Model file for the job. Use its own axes, mm. A direction names the side the tool comes from. Give positions to 0.01 mm unless a question says otherwise; leave off trailing zeros. Write each loop counter-clockwise with the first axis right and the second up, starting at its lowest first coordinate (ties: lowest second). Pieces come first, ordered by that corner, then holes. Notation, with made-up numbers: M 54,31.25 L 89,31.25 A32 cw 89,57.25 Z; hole C -11,50 d3. An arc over 180 degrees is marked long. Answer as a JSON object with one key per item and string values. Group by question number.
```python
from build123d import *

# Parameters (mm, degrees)
BOSS_EXTRUDE1_DEPTH = 9.5
SKETCH3_R           = 2.75
SKETCH3_R_2         = 1.25
CUT_EXTRUDE1_DEPTH  = 19.054661658


with BuildPart() as part:
    # Sketch2 → Boss-Extrude1 (new body, symmetric)
    with BuildSketch(Plane.XY):
        with BuildLine():
            Line((-37.204062484, 20.661621188), (-37.204062484, 2.661621188))
            ThreePointArc((-37.204062484, 2.661621188), (-35.886988122, -0.518077598), (-32.707289335, -1.83515196))
            Line((-32.707289335, -1.83515196), (-22.999692171, -1.83515196))
            ThreePointArc((-22.999692171, -1.83515196), (-20.057423766, -0.468366217), (-19.204062484, 2.661621188))
            Line((-19.204062484, 2.661621188), (-19.204062484, 20.661621188))
            Line((-19.204062484, 20.661621188), (-37.204062484, 20.661621188))
        make_face()
    extrude(amount=BOSS_EXTRUDE1_DEPTH, both=True)

    # Sketch3 → Cut-Extrude1 (cut, through all)
    with BuildSketch(Plane.ZY.offset(37.204062484)):
        with Locations((0, 11.661621188)):
            Circle(SKETCH3_R)
        with Locations((6.125, 11.661621188)):
            Circle(SKETCH3_R_2)
        with Locations((-6.125, 11.661621188)):
            Circle(SKETCH3_R_2)
    extrude(amount=-CUT_EXTRUDE1_DEPTH, mode=Mode.SUBTRACT)


solid = part.part
```
Q1. Wall check: L1, parallel to Z at x = -33.75, y = 10.75; L2, parallel to Z at x = -31.5, y = 11; L3, parallel to X at y = 11, z = 2.75. Give the ranges that are in metal, low to high.
Q2. 3-axis set-ups, long thin cutter, end or side, ignore diameter. For faces 4 (the flat face through (-28, 10, 9.5)), 5 (the flat face through (-19.204, 9.5, 2.2)): which of +Z, -Z, +X, -X, +Y, -Y reach the whole face in a straight line?
Q3. Slice it at C-C, the plane y = 12.5. Write the cut outline in (x, z).
Q4. Two-plate mould, pull along Z, no slides. Class faces 1 (the cylindrical face through (-20.088, -0.504, 0.133)), 2 (the flat face through (-28, 10, -9.5)), 3 (the cylindrical face through (-28.33, 8.977, -0.596)): +Z half, -Z half, draft (parallel to the pull), parting line (faces both ways), or undercut.
Q5. Slice it at B-B, the plane x = -20.25. Write the cut outline in (y, z) (3 decimals), then the cut area to 3 significant figures.
Q6. Drop flat-ended pins along their axis: P1, Ø3, axis at y = 11.66, z = -6.12, coming from the +X side; P2, Ø2, axis at y = 11.66, z = 6.12, coming from the -X side. Give the stop position or say it passes through.
Q7. Slice it at A-A, the plane z = 0. Write the cut outline in (x, y).
Q8. Slice it at D-D, the plane z = -8. Write the cut outline in (x, y), then the cut area to 3 significant figures.
Solved:
{
 "1": {"L1": "z = -9.5 to -6.98, -5.27 to -2.59, 2.59 to 5.27, 6.98 to 9.5", "L2": "z = -9.5 to -7.19, -5.06 to -2.67, 2.67 to 5.06, 7.19 to 9.5", "L3": "x = -37.2 to -19.2"},
 "2": {"face 4": "+Z, +X, -X, +Y, -Y", "face 5": "+Z, -Z, +X, +Y"},
 "3": {"outline": "M -37.2,-9.5 L -19.2,-9.5 L -19.2,-7.05 L -37.2,-7.05 Z; M -37.2,-5.2 L -19.2,-5.2 L -19.2,-2.62 L -37.2,-2.62 Z; M -37.2,2.62 L -19.2,2.62 L -19.2,5.2 L -37.2,5.2 Z; M -37.2,7.05 L -19.2,7.05 L -19.2,9.5 L -37.2,9.5 Z"},
 "4": {"face 1": "draft", "face 2": "-Z half", "face 3": "undercut"},
 "5": {"outline": "M -0.68,-9.5 L 20.662,-9.5 L 20.662,9.5 L -0.68,9.5 Z; hole C 11.662,0 d5.5; hole C 11.662,-6.125 d2.5; hole C 11.662,6.125 d2.5", "area": "372 mm²"},
 "6": {"P1": "stops at x = -19.2", "P2": "passes through"},
 "7": {"outline": "M -37.2,2.66 A4.5 ccw -32.71,-1.84 L -23,-1.84 A3.85 ccw -19.2,2.66 L -19.2,8.91 L -37.2,8.91 Z; M -37.2,14.41 L -19.2,14.41 L -19.2,20.66 L -37.2,20.66 Z"},
 "8": {"outline": "M -37.2,2.66 A4.5 ccw -32.71,-1.84 L -23,-1.84 A3.85 ccw -19.2,2.66 L -19.2,20.66 L -37.2,20.66 Z", "area": "398 mm²"}
}
